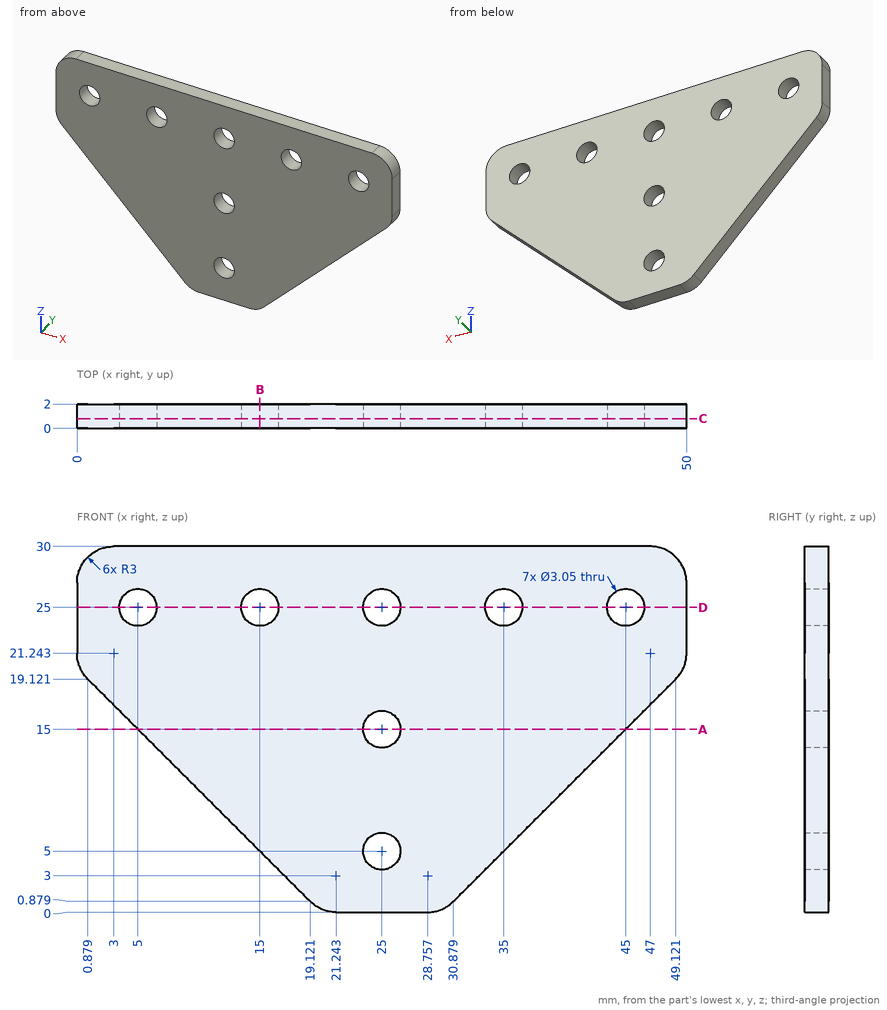
Job drawing, mm, ordinate dimensions from the low corner. One solid piece. Coordinates: 2 decimals unless noted, no trailing zeros. Order: outer loops, then holes, each group sorted by start corner. A loop starts at its lowest first (then second) coordinate and runs counter-clockwise, first axis right, second up. Notation, with made-up numbers: (16.5, 42.5) -> (41.5, 42.5) arc R20 ccw to (41.5, 51.5) -> close; hole circle Ø8 at (-12, 21.5). An arc over 180 degrees is marked (long way). Put each result on its own line as item: value. Start each with the question number.
(1) Band-saw the part on C-C (y = 0.8). Count the separate pieces of the cut face and the enclosed holes in it, then the cut area to 3 significant figures.
(2) Pin check, flat tips, straight feed: pin 1 Ø3.5 at (x, z) = (25, 5) entering from -Y; pin 2 Ø2.5 at (x, z) = (25, 25) entering from -Y. Stop position of each tip, or through.
(3) Band-saw the part on D-D (z = 25). Give the cut face in (x, y) (1 decimal).
(4) Probe line 1 along X through (y, z) = (0.55, 25) (1 decimal); line 2 along Z through (x, y) = (46, 0.75); line 3 along Z through (x, y) = (6, 1.45). List the from-to ranges inside material, lowest first. Write a range as [from, to].
(5) Band-saw the part on B-B (x = 15). Give the cut face in (y, z) (1 decimal), then the cut area to 3 significant figures.
(6) Band-saw the part on A-A (z = 15). Give the cut face in (x, y) (1 decimal).
Determined:
1. separate pieces: 1
1. enclosed holes: 7
1. area: 1,040 mm²
2. pin 1: stops at y = 0
2. pin 2: passes through
3. outline: (0, 0) -> (3.5, 0) -> (3.5, 2) -> (0, 2) -> close; (6.5, 0) -> (13.5, 0) -> (13.5, 2) -> (6.5, 2) -> close; (16.5, 0) -> (23.5, 0) -> (23.5, 2) -> (16.5, 2) -> close; (26.5, 0) -> (33.5, 0) -> (33.5, 2) -> (26.5, 2) -> close; (36.5, 0) -> (43.5, 0) -> (43.5, 2) -> (36.5, 2) -> close; (46.5, 0) -> (50, 0) -> (50, 2) -> (46.5, 2) -> close
4. line 1: x = [0, 3.5], [6.5, 13.5], [16.5, 23.5], [26.5, 33.5], [36.5, 43.5], [46.5, 50]
4. line 2: z = [16, 23.85], [26.15, 30]
4. line 3: z = [14, 23.85], [26.15, 30]
5. outline: (0, 5) -> (2, 5) -> (2, 23.5) -> (0, 23.5) -> close; (0, 26.5) -> (2, 26.5) -> (2, 30) -> (0, 30) -> close
5. area: 43.9 mm²
6. outline: (5, 0) -> (23.5, 0) -> (23.5, 2) -> (5, 2) -> close; (26.5, 0) -> (45, 0) -> (45, 2) -> (26.5, 2) -> close
